Model file for the job. Use its own axes, mm. A direction names the side the tool comes from. Give positions to 0.01 mm unless a question says otherwise; leave off trailing zeros. Loops run counter-clockwise (first coordinate to the right, second up) from the corner with the lowest first, then second, coordinate; pieces in that order, holes last. Notation, with made-up numbers: M -36.5,69.25 L -27.5,69.25 A19 ccw -27.5,73.25 Z; hole C 64.25,26 d4. An arc over 180 degrees is marked long. Answer in a Markdown table with one row per item.
Autodesk Inventor part; units mm, degrees
ref_plane "YZ Plane" through (0, 0, 0) normal (1, 0, 0) x (0, 1, 0)
ref_plane "XZ Plane" through (0, 0, 0) normal (0, 1, 0) x (-1, 0, 0)
ref_plane "XY Plane" through (0, 0, 0) normal (0, 0, 1) x (1, 0, 0)
sketch "Sketch4" plane through (0, 0, 0) normal (0, 0, 1) x (1, 0, 0)
  arc A0 (2.5, 0) -> (2.5, -10.2) centre (6.452, -5.1) ccw
  arc A1 (9.7, -10.2) -> (9.7, 0) centre (5.748, -5.1) ccw
  line L0 (-2, 2) -> (14.2, 2)
  line L1 (14.2, 2) -> (14.2, -10.2)
  line L2 (-2, -10.2) -> (-2, 2)
  line L3 (-2, -10.2) -> (2.5, -10.2)
  line L4 (9.7, -10.2) -> (14.2, -10.2)
  line L5 (2.5, 0) -> (9.7, 0)
  point P0 (0, 0)
  point P1 (6.1, 0)
  point P2 (6.1, -10.2)
  dimension "d50" = 3.6
  dimension "d51" = 3.6
  dimension "d52" = 3.6
  dimension "d53" = 3.6
extrude "Extrusion4" add sketch "Sketch4" along normal blind 15
ref_plane "Work Plane2" through (6.1, -10.2, 0) normal (1, 0, 0) x (0, 0, -1)
sketch "Sketch5" plane through (6.1, -10.2, 0) normal (1, 0, 0) x (0, 0, -1)
  line L0 (0, 0) -> (0, 12.2)
  line L1 (0, 12.2) -> (-15, 12.2)
  line L2 (-15, 0) -> (-15, 12.2)
  line L3 (0, 0) -> (-15, 0)
  line L4 (1, 0) -> (-21.5, 0)
  line L5 (-21.5, 0) -> (-21.5, -22.5)
  line L6 (-21.5, -22.5) -> (1, -22.5)
  line L7 (1, -22.5) -> (1, 0)
  line L8 (-20.5, -1) -> (0, -1)
  line L9 (0, -21.5) -> (-20.5, -21.5)
  line L10 (-20.5, -8.25) -> (-14.5, -8.25)
  line L11 (-14.5, -8.25) -> (-14.5, -14.25)
  line L12 (-14.5, -14.25) -> (-20.5, -14.25)
  line L13 (0, -8.25) -> (-6, -8.25)
  line L14 (-6, -8.25) -> (-6, -14.25)
  line L15 (-6, -14.25) -> (0, -14.25)
  line L16 (-20.5, -21.5) -> (-20.5, -14.25)
  line L17 (-20.5, -8.25) -> (-20.5, -1)
  line L18 (0, -1) -> (0, -8.25)
  line L19 (0, -14.25) -> (0, -21.5)
  point P0 (0, 10.2)
  point P1 (-20.5, -11.25)
  point P2 (-20.5, -11.25)
  dimension "d58" = 22.5
  dimension "d59" = 22.5
  dimension "d60" = 1
  dimension "d61" = 1
extrude "Extrusion5" add sketch "Sketch5" along normal mid plane 30 contours L4 L7 L6 L5 L3
sketch "Sketch6" plane through (-8.9, -10.2, 21.5) normal (0, 1, 0) x (1, 0, 0)
  circle A0 centre (3.5, 11.25) radius 2.5
  line L0 (0, 0) -> (0, 22.5)
  point P0 (8.9, 21.5)
  dimension "d69" = 5
  dimension "d70" = 3.5
extrude "Extrusion6" cut sketch "Sketch6" along normal through all both and the other way through all
properties part number "motor mount left"
(1) Flat gauge pins, fed straight in: P1, Ø12, axis at x = -4.5, y = -4, coming from the -Z side; P2, Ø10, axis at x = 4, y = -3, coming from the +Z side; P3, Ø3, axis at y = -6.5, z = 9.5, coming from the +X side. Where does each tip first touch, or does it go through?
Established:
| item | result |
|---|---|
| P1 | stops at z = 0 |
| P2 | stops at z = 15 |
| P3 | stops at x = 14.2 |
(2) Which spindle directions (+Z, -Z, +X, -X, +Y, -Y) get a long thin tool onto all of the face, cutting with end or side? Do faces 1 (the flat face through (-2, -4, 7)), 2 (the flat face through (6, 1, 15)), 3 (the flat face through (6, -21, 6)), 4 (the cylindrical face through (12.2, -5, 7.4)). Say none if no direction does.
Established:
| item | result |
|---|---|
| face 1 | +Z, -Z, -X, +Y |
| face 2 | +Z, +X, -X, +Y |
| face 3 | +X, -X |
| face 4 | +Z, -Z |
(3) Wall check: L1, parallel to Y at x = 2.5, z = 14.75; L2, parallel to Y at x = 12, z = 19.5; L3, parallel to Y at x = 14, z = 3.75. Give the ranges that are in metal, low to high.
Established:
| item | result |
|---|---|
| L1 | y = -32.7 to -31.7, -24.45 to -18.45, -11.2 to -10.2, 0 to 2 |
| L2 | y = -32.7 to -31.7, -24.45 to -18.45, -11.2 to -10.2 |
| L3 | y = -32.7 to -31.7, -24.45 to -18.45, -11.2 to 2 |
(4) Mould opens along Y. For faces 5 (the flat face through (6, -28, 0)), 6 (the flat face through (6, -22, -1)), 7 (the flat face through (6, 2, 7)), 8 (the flat face through (6, -15, 0)) say: pulls with the +Y half, pulls with the -Y half, needs draft (parallel to the pull), parting line crosses it, or undercut.
Established:
| item | result |
|---|---|
| face 5 | undercut |
| face 6 | needs draft |
| face 7 | pulls with the +Y half |
| face 8 | undercut |
(5) Saw through at D-D, the plane z = 5.5. Give the cut face in (x, y).
Established:
| item | result |
|---|---|
| outline | M -8.9,-32.7 L 21.1,-32.7 L 21.1,-31.7 L -8.9,-31.7 Z; M -8.9,-24.45 L 21.1,-24.45 L 21.1,-18.45 L -8.9,-18.45 Z; M -8.9,-11.2 L 21.1,-11.2 L 21.1,-10.2 L 14.2,-10.2 L 14.2,2 L -2,2 L -2,-10.2 L -8.9,-10.2 Z; hole M 2.5,-10.2 L 9.7,-10.2 A6.45 ccw 9.7,0 L 2.5,0 A6.45 ccw Z |
(6) Saw through at C-C, the plane y = -28. Give the cut face in (x, z), and give its area (3 significant figures).
Established:
| item | result |
|---|---|
| outline | M -8.9,-1 L 21.1,-1 L 21.1,0 L -8.9,0 Z; M -8.9,20.5 L 21.1,20.5 L 21.1,21.5 L -8.9,21.5 Z |
| area | 60.0 mm2 |
(7) Saw through at B-B, the plane x = 17. Give the cut face in (y, z), and give its area (3 significant figures).
Established:
| item | result |
|---|---|
| outline | M -32.7,-1 L -10.2,-1 L -10.2,21.5 L -32.7,21.5 Z; hole M -31.7,0 L -24.45,0 L -24.45,6 L -18.45,6 L -18.45,0 L -11.2,0 L -11.2,20.5 L -18.45,20.5 L -18.45,14.5 L -24.45,14.5 L -24.45,20.5 L -31.7,20.5 Z |
| area | 158 mm2 |
(8) Saw through at A-A, the plane z = 8.25. Give the cut face in (x, y), and give its area (3 significant figures).
Established:
| item | result |
|---|---|
| outline | M -8.9,-32.7 L -6.9,-32.7 L -6.9,-31.7 L -8.9,-31.7 Z; M -8.9,-11.2 L -6.9,-11.2 L -6.9,-10.2 L -8.9,-10.2 Z; M -3.9,-32.7 L 21.1,-32.7 L 21.1,-31.7 L -3.9,-31.7 Z; M -3.9,-11.2 L 21.1,-11.2 L 21.1,-10.2 L 14.2,-10.2 L 14.2,2 L -2,2 L -2,-10.2 L -3.9,-10.2 Z; hole M 2.5,-10.2 L 9.7,-10.2 A6.45 ccw 9.7,0 L 2.5,0 A6.45 ccw Z |
| area | 143 mm2 |
